Can you work these out from the model? Positions are in its coordinate system, mm. Face numbers are marked on the shaded views. A direction names the side the tool comes from. Round coordinates to 2 decimals unless told otherwise and drop trailing zeros. Order: outer loops, then holes, each group sorted by start corner. A loop starts at its lowest first (then second) coordinate and runs counter-clockwise, first axis right, second up. Notation, with made-up numbers: (-2.75, 19) - (50.25, 19) arc R37 cw to (50.25, 57) - close; hole circle Ø7 at (-15.5, 16). An arc over 180 degrees is marked (long way). Write item = value, one per line.
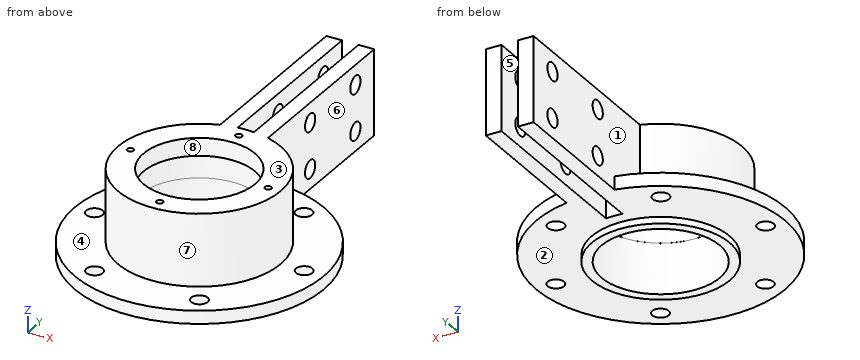
from build123d import *

# Parameters (mm, degrees)
SKETCH1_R              = 42.5
BOSS_EXTRUDE1_DEPTH    = 65
SKETCH2_R              = 42.5
BOSS_EXTRUDE2_DEPTH    = 10
SKETCH3_R              = 45.05
CUT_EXTRUDE1_DEPTH     = 33.5
SKETCH4_R              = 44.9925
CUT_EXTRUDE2_DEPTH     = 18
F_12_0MM_DOWEL_HOLE1_D = 12.5
M6_TAPPED_HOLE1_D      = 5
M6_TAPPED_HOLE1_DEPTH  = 12
M6_TAPPED_HOLE1_TIP    = 1.502151548
BOSS_EXTRUDE3_START    = 5
SKETCH10_R             = 52.5
SKETCH10_R_2           = 45.05
BOSS_EXTRUDE3_DEPTH    = 5
F_12_0MM_DOWEL_HOLE2_D = 13.5


with BuildPart() as part:
    # Sketch1 → Boss-Extrude1 (new body)
    with BuildSketch(Plane.XY):
        with BuildLine():
            Line((-18.25, 59.253164472), (-18.25, 200.253164472))
            Line((-18.25, 200.253164472), (-6.25, 200.253164472))
            Line((-6.25, 200.253164472), (-6.25, 61.684175442))
            ThreePointArc((-6.25, 61.684175442), (0, 62), (6.25, 61.684175442))
            Line((6.25, 61.684175442), (6.25, 200.253164472))
            Line((6.25, 200.253164472), (18.25, 200.253164472))
            Line((18.25, 200.253164472), (18.25, 59.253164472))
            ThreePointArc((18.25, 59.253164472), (0, -62), (-18.25, 59.253164472))
        make_face()
        Circle(SKETCH1_R, mode=Mode.SUBTRACT)
    extrude(amount=BOSS_EXTRUDE1_DEPTH)

    # Sketch2 → Boss-Extrude2 (add)
    # profile 1 of 2: a face of its own
    with BuildSketch(Plane(origin=(0, 0, 0), x_dir=(-1, 0, 0), z_dir=(0, 0, -1))):
        with BuildLine():
            ThreePointArc((-18.25, 93.230560977), (0, -95), (18.25, 93.230560977))
            Line((18.25, 93.230560977), (18.25, 59.253164472))
            ThreePointArc((18.25, 59.253164472), (0, -62), (-18.25, 59.253164472))
            Line((-18.25, 59.253164472), (-18.25, 93.230560977))
        make_face()
    # profile 2 of 2: a face of its own
    with BuildSketch(Plane(origin=(0, 0, 0), x_dir=(-1, 0, 0), z_dir=(0, 0, -1))):
        with BuildLine():
            ThreePointArc((18.25, 93.230560977), (12.27492281, 94.203642552), (6.25, 94.794184948))
            Line((6.25, 94.794184948), (6.25, 61.684175442))
            ThreePointArc((6.25, 61.684175442), (0, 62), (-6.25, 61.684175442))
            Line((-6.25, 61.684175442), (-6.25, 94.794184948))
            ThreePointArc((-6.25, 94.794184948), (-12.27492281, 94.203642552), (-18.25, 93.230560977))
            Line((-18.25, 93.230560977), (-18.25, 59.253164472))
            ThreePointArc((-18.25, 59.253164472), (0, -62), (18.25, 59.253164472))
            Line((18.25, 59.253164472), (18.25, 93.230560977))
        make_face()
        with Locations(Location((0, 0, 0), (0, 0, 180))):
            Circle(SKETCH2_R, mode=Mode.SUBTRACT)
    extrude(amount=-BOSS_EXTRUDE2_DEPTH)

    # Sketch3 → Cut-Extrude1 (cut)
    with BuildSketch(Plane(origin=(0, 0, 0), x_dir=(-1, 0, 0), z_dir=(0, 0, -1))):
        Circle(SKETCH3_R)
    extrude(amount=-CUT_EXTRUDE1_DEPTH, mode=Mode.SUBTRACT)

    # Sketch4 → Cut-Extrude2 (cut)
    with BuildSketch(Plane(origin=(0, 0, 33.5), x_dir=(-1, 0, 0), z_dir=(0, 0, -1))):
        Circle(SKETCH4_R)
    extrude(amount=-CUT_EXTRUDE2_DEPTH, mode=Mode.SUBTRACT)

    # Ø12.0mm Dowel Hole1 (through all)
    with Locations(Plane(origin=(0, 0, 0), x_dir=(-1, 0, 0), z_dir=(0, 0, -1))):
        with Locations((-40, -69.282032303), (-80, 0), (-40, 69.282032303), (40, 69.282032303), (80, 0), (40, -69.282032303)):
            Hole(F_12_0MM_DOWEL_HOLE1_D / 2)

    # M6 Tapped Hole1
    with Locations(Plane.XY.offset(65)):
        with Locations((0, -52.5), (-52.5, 0), (0, 52.5), (52.5, 0)):
            Hole(M6_TAPPED_HOLE1_D / 2, depth=M6_TAPPED_HOLE1_DEPTH)
            with Locations((0, 0, -(M6_TAPPED_HOLE1_DEPTH + M6_TAPPED_HOLE1_TIP / 2))):  # 118° drill point
                Cone(0, M6_TAPPED_HOLE1_D / 2, M6_TAPPED_HOLE1_TIP, mode=Mode.SUBTRACT)

    # Sketch10 → Boss-Extrude3 (add)
    with BuildSketch(Plane(origin=(0, 0, 0), x_dir=(-1, 0, 0), z_dir=(0, 0, -1)).offset(BOSS_EXTRUDE3_START)):
        with Locations(Location((0, 0, 0), (0, 0, 180))):
            Circle(SKETCH10_R)
        Circle(SKETCH10_R_2, mode=Mode.SUBTRACT)
    extrude(amount=-BOSS_EXTRUDE3_DEPTH)

    # Ø12.0mm Dowel Hole2 (through all)
    with Locations(Plane.ZY.offset(18.25)):
        with Locations((15, 175.253164472), (50, 175.253164472), (50, 115.253164472), (15, 115.253164472)):
            Hole(F_12_0MM_DOWEL_HOLE2_D / 2)


solid = part.part
(1) On a 3-axis mill with a long thin cutter (end or side, diameter ignored), from which of +Z, -Z, +X, -X, +Y, -Y can I reach the whole of each face in a straight line? I mean the marked faces 1, 2, 3, 4 and 5. Say none if no direction works.
Computed:
face_1 = +Z, -X, +Y
face_2 = -Z
face_3 = +Z, +X, -X, +Y, -Y
face_4 = +Z
face_5 = +Z, -Z, +Y
(2) If we section it at B-B (x = -14): Write out the boundary of the cut face in (y, z).
Computed:
outline = (-93.96, 0) - (-50.6, 0) - (-50.6, -5) - (-42.82, -5) - (-42.82, 33.5) - (-42.76, 33.5) - (-42.76, 51.5) - (-40.13, 51.5) - (-40.13, 65) - (-60.4, 65) - (-60.4, 10) - (-93.96, 10) - close; (40.13, 51.5) - (42.76, 51.5) - (42.76, 33.5) - (42.82, 33.5) - (42.82, -5) - (50.6, -5) - (50.6, 0) - (200.25, 0) - (200.25, 65) - (40.13, 65) - close; hole circle Ø13.5 at (115.25, 15); hole circle Ø13.5 at (115.25, 50); hole circle Ø13.5 at (175.25, 15); hole circle Ø13.5 at (175.25, 50)
(3) Will these pins go through, and if not, where does the flat tip stop? P1, Ø17.5, axis at y = 115.25, z = 50, coming from the -X side; P2, Ø10, axis at x = -44, z = 53, coming from the -Y side; P3, Ø4, axis at x = 52.5, y = 0, coming from the +Z side; P4, Ø7.5, axis at x = -40, y = -69.28, coming from the +Z side.
Computed:
P1 = -18.25
P2 = -48.2
P3 = 52.7
P4 = through
(4) If we section it at C-C (y = 37): Write out the boundary of the cut face in (x, z), plus the area to 3 significant figures.
Computed:
outline = (-87.5, 0) - (-37.25, 0) - (-37.25, -5) - (-25.7, -5) - (-25.7, 33.5) - (-25.6, 33.5) - (-25.6, 51.5) - (-20.91, 51.5) - (-20.91, 65) - (-49.75, 65) - (-49.75, 10) - (-87.5, 10) - close; (20.91, 51.5) - (25.6, 51.5) - (25.6, 33.5) - (25.7, 33.5) - (25.7, -5) - (37.25, -5) - (37.25, 0) - (87.5, 0) - (87.5, 10) - (49.75, 10) - (49.75, 65) - (20.91, 65) - close
area = 4,130 mm^2
(5) If we section it at A-A (z = 15): Write out the boundary of the cut face in (x, y), plus the area to 3 significant figures.
Computed:
outline = (-18.25, 59.25) arc R62 ccw (long way) to (18.25, 59.25) - (18.25, 108.5) - (6.25, 108.5) - (6.25, 61.68) arc R62 ccw to (-6.25, 61.68) - (-6.25, 108.5) - (-18.25, 108.5) - close; (-18.25, 122) - (-6.25, 122) - (-6.25, 168.5) - (-18.25, 168.5) - close; (-18.25, 182) - (-6.25, 182) - (-6.25, 200.25) - (-18.25, 200.25) - close; (6.25, 122) - (18.25, 122) - (18.25, 168.5) - (6.25, 168.5) - close; (6.25, 182) - (18.25, 182) - (18.25, 200.25) - (6.25, 200.25) - close; hole circle Ø90.1 at (0, 0)
area = 8,400 mm^2
(6) If we section it at D-D (z = 30.5): Write out the boundary of the cut face in (x, y), plus the area to 3 significant figures.
Computed:
outline = (-18.25, 59.25) arc R62 ccw (long way) to (18.25, 59.25) - (18.25, 200.25) - (6.25, 200.25) - (6.25, 61.68) arc R62 ccw to (-6.25, 61.68) - (-6.25, 200.25) - (-18.25, 200.25) - close; hole circle Ø90.1 at (0, 0)
area = 9,050 mm^2
(7) If I drill on line 1 (Y direction, x = 0, z = 57); line 2 (Y direction, x = -14.5, z = 17.5); line 3 (X direction, y = 171.5, z = 61), over which ranges is the centre line in solid material (lowest first)? Write a range as from..to.
Computed:
line_1 = -62..-55, -50..-42.5, 42.5..50, 55..62
line_2 = -60.28..-42.65, 42.65..108.98, 121.52..168.98, 181.52..200.25
line_3 = -18.25..-6.25, 6.25..18.25
(8) Thinking about a two-plate mould opening in Y: for the marked faces 6, 7 and 8, which applies, +Y half, -Y half, draft (parallel to the pull), parting line (faces both ways), or undercut?
Computed:
face_6 = draft
face_7 = parting line
face_8 = undercut
